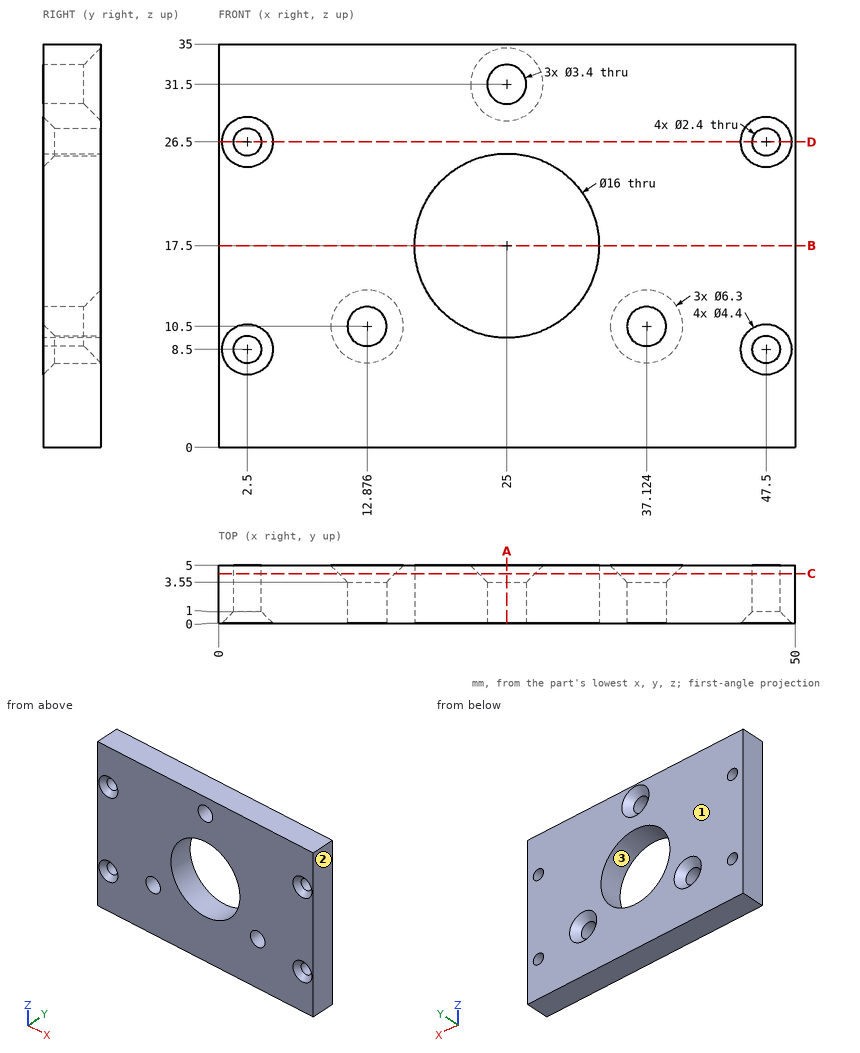
For this review, use the dimensioned drawing (mm, ordinates from the lowest corner) and the shaded views. Give positions to 0.01 mm unless a question says otherwise; leave off trailing zeros. Loops run counter-clockwise (first coordinate to the right, second up) from the corner with the lowest first, then second, coordinate; pieces in that order, holes last. Notation, with made-up numbers: (33.5, -28.75) -> (78.5, -28.75) arc R20 ccw to (78.5, -3.75) -> close; hole circle Ø5 at (-5.5, 85.25). An arc over 180 degrees is marked (long way). One line per question, with ' | ' between items. Start each with the question number.
(1) For line 1 (X direction, y = 2, z = 8.5); line 2 (Z direction, x = 47.5, y = 4.15); line 3 (X direction, y = 4, z = 17.5), list the stretches that pass through material, from the lowest coordinate up.
(2) We need section C-C (y = 4.3). State how many separate pieces and enclosed holes the cut face has, and give its area (3 significant figures).
(3) We need section A-A (x = 25). State the section outline as (y, z) points.
(4) Draft analysis for pull direction X (two halves, no side actions). For the marked faces 1, 2 and 3, state which applies: +X half, -X half, draft (parallel to the pull), parting line (faces both ways), or undercut.
(5) We need section D-D (z = 26.5). State the section outline as (x, y) points, and give its area (3 significant figures).
(6) We need section B-B (z = 17.5). State the section outline as (x, y) points.
(7) Insertion check: P1, Ø1.4, axis at x = 47.5, z = 8.5, coming from the -Y side; P2, Ø1, axis at y = 0.5, z = 6.5, coming from the -X side; P3, Ø5.5, axis at x = 25, z = 31.5, coming from the +Y side. Each pin has a flat end and moves straight along its axis. Give the tip position at first contact, or say it passes through.
The answers:
1) line 1: x = 0 to 1.3, 3.7 to 46.3, 48.7 to 50 | line 2: z = 0 to 7.3, 9.7 to 25.3, 27.7 to 35 | line 3: x = 0 to 17, 33 to 50
2) separate pieces: 1 | enclosed holes: 8 | area: 1,470 mm^2
3) outline: (0, 0) -> (5, 0) -> (5, 9.5) -> (0, 9.5) -> close; (0, 25.5) -> (5, 25.5) -> (5, 28.35) -> (3.55, 29.8) -> (0, 29.8) -> close; (0, 33.2) -> (3.55, 33.2) -> (5, 34.65) -> (5, 35) -> (0, 35) -> close
4) face 1: draft | face 2: +X half | face 3: undercut
5) outline: (0, 0) -> (0.3, 0) -> (1.3, 1) -> (1.3, 5) -> (0, 5) -> close; (3.7, 1) -> (4.7, 0) -> (45.3, 0) -> (46.3, 1) -> (46.3, 5) -> (3.7, 5) -> close; (48.7, 1) -> (49.7, 0) -> (50, 0) -> (50, 5) -> (48.7, 5) -> close | area: 224 mm^2
6) outline: (0, 0) -> (17, 0) -> (17, 5) -> (0, 5) -> close; (33, 0) -> (50, 0) -> (50, 5) -> (33, 5) -> close
7) P1: passes through | P2: stops at x = 0 | P3: stops at y = 4.6
